Could you check a few things on this model? Use its own coordinates, in mm. A direction names the side the tool comes from. Coordinates: 2 decimals unless noted, no trailing zeros. Order: outer loops, then holes, each group sorted by start corner. A loop starts at its lowest first (then second) coordinate and runs counter-clockwise, first axis right, second up. Notation, with made-up numbers: (21, 73) -> (34, 73) arc R23 cw to (34, 92) -> close; hole circle Ø8 at (25.5, 38.25). An arc over 180 degrees is marked (long way). Put each result on its own line as item: value. Start each with the question number.
Q1. Please list where these lines run through material, in increasing order: line 1 along X through (y, z) = (24.5, 0.25); line 2 along Z through (x, y) = (-1.25, 20.5); line 3 along X through (y, z) = (14, 2.5).
Q2. Will these pins go through, and if not, where does the flat tip stop? pin 1 (1.5 mm diameter, centred on y = 36.5, z = 1.5, fed in from +X); pin 2 (3 mm diameter, centred on x = -1, y = 19.5, fed in from +Z) (3 decimals); pin 3 (3 mm diameter, centred on x = -2, y = 36, fed in from +Z) (3 decimals); pin 4 (1.5 mm diameter, centred on y = 26.5, z = -1, fed in from +X).
Q3. If we section it at C-C (y = 35.5): Please give me the cut outline in (x, z), and give its area (3 significant figures).
Q4. For faces 1 (the face through (2, 25.4, -2)), 2 (the face through (1.93, 12.52, 2.52)), which set-ups out of +Z, -Z, +X, -X, +Y, -Y let a thin tool reach every point of the face, with its end or its side?
Q5. If we section it at B-B (z = 0): Please give me the cut outline in (x, y) (3 decimals).
Q6. If we section it at A-A (x = 0): Please give me the cut outline in (y, z) (3 decimals), and give its area (3 significant figures).
Q7. If we section it at D-D (y = 12): Please give me the cut outline in (x, z) (3 decimals), and give its area (3 significant figures).
from build123d import *

# Parameters (mm, degrees)
SKETCH1_R           = 3.175
BOSS_EXTRUDE1_DEPTH = 38.1
SKETCH2_R           = 3.591307694
SKETCH2_R_2         = 2.3
CUT_EXTRUDE1_DEPTH  = 12.7
SKETCH3_R           = 1.984375
BOSS_EXTRUDE2_DEPTH = 12.7


with BuildPart() as part:
    # Sketch1 → Boss-Extrude1 (new body)
    with BuildSketch(Plane(origin=(0, 0, 0), x_dir=(1, 0, 0), z_dir=(0, 1, 0))):
        with Locations(Location((0, 0, 0), (0, 0, 90))):
            Circle(SKETCH1_R)
    extrude(amount=BOSS_EXTRUDE1_DEPTH)

    # Sketch2 → Cut-Extrude1 (cut)
    with BuildSketch(Plane(origin=(0, 38.1, 0), x_dir=(1, 0, 0), z_dir=(0, 1, 0))):
        Circle(SKETCH2_R)
        with Locations(Location((0, 0, 0), (0, 0, 270))):
            Circle(SKETCH2_R_2, mode=Mode.SUBTRACT)
    extrude(amount=-CUT_EXTRUDE1_DEPTH, mode=Mode.SUBTRACT)

    # Sketch3 → Boss-Extrude2 (add)
    with BuildSketch(Plane(origin=(0, 38.1, 0), x_dir=(1, 0, 0), z_dir=(0, 1, 0))):
        with Locations(Location((0, 0, 0), (0, 0, 270))):
            Circle(SKETCH3_R)
    extrude(amount=BOSS_EXTRUDE2_DEPTH)


solid = part.part
The answers:
1. line 1: -3.17 to 3.17
1. line 2: -2.92 to 2.92
1. line 3: -1.96 to 1.96
2. pin 1: x = 2.17
2. pin 2: z = 3.175
2. pin 3: z = 2.245
2. pin 4: x = 2.29
3. outline: circle Ø4.6 at (0, 0)
3. area: 16.6 mm^2
4. face 1: +Y
4. face 2: +Y, -Y
5. outline: (-3.175, 0) -> (3.175, 0) -> (3.175, 25.4) -> (2.3, 25.4) -> (2.3, 38.1) -> (1.984, 38.1) -> (1.984, 50.8) -> (-1.984, 50.8) -> (-1.984, 38.1) -> (-2.3, 38.1) -> (-2.3, 25.4) -> (-3.175, 25.4) -> close
6. outline: (0, -3.175) -> (25.4, -3.175) -> (25.4, -2.3) -> (38.1, -2.3) -> (38.1, -1.984) -> (50.8, -1.984) -> (50.8, 1.984) -> (38.1, 1.984) -> (38.1, 2.3) -> (25.4, 2.3) -> (25.4, 3.175) -> (0, 3.175) -> close
6. area: 270 mm^2
7. outline: circle Ø6.35 at (0, 0)
7. area: 31.7 mm^2
